from build123d import *

# Parameters (mm, degrees)
SKETCH_1_R           = 15
SKETCH_1_R_2         = 1.1
EXTRUDE_1_DEPTH      = 8
EXTRUDE_2_DEPTH      = 22
EXTRUDE_2_DEPTH_BACK = 22
SKETCH_5_W           = 12.455474759
SKETCH_5_H           = 13.140065833
CUT_EXTRUDE_1_DEPTH  = 15
CUT_EXTRUDE_START    = -15
CUT_EXTRUDE_2_DEPTH  = 15
SKETCH_7_R           = 4
EXTRUDE_3_DEPTH      = 2
SKETCH_8_R           = 3
CUT_EXTRUDE_3_DEPTH  = 1
DOME_1_FACE_RADIUS   = 3
DOME_1_HEIGHT        = 1.5
FILLET_1_R           = 3


with BuildPart() as part:
    # 草图1 → 凸台-拉伸1 (new body)
    with BuildSketch(Plane.XY):
        with BuildLine():
            Line((13.964240044, -17), (-13.964240044, -17))
            ThreePointArc((-13.964240044, -17), (-22, 0), (-13.964240044, 17))
            Line((-13.964240044, 17), (13.964240044, 17))
            ThreePointArc((13.964240044, 17), (22, 0), (13.964240044, -17))
        make_face()
        Circle(SKETCH_1_R, mode=Mode.SUBTRACT)
        with Locations((-13, 12)):
            Circle(SKETCH_1_R_2, mode=Mode.SUBTRACT)
        with Locations((13, 12)):
            Circle(SKETCH_1_R_2, mode=Mode.SUBTRACT)
        with Locations((13, -12)):
            Circle(SKETCH_1_R_2, mode=Mode.SUBTRACT)
        with Locations((-13, -12)):
            Circle(SKETCH_1_R_2, mode=Mode.SUBTRACT)
    extrude(amount=EXTRUDE_1_DEPTH)

    # 草图3 → 凸台-拉伸2 (add, two sides: drawn at the far end of the back side and taken through both)
    with BuildSketch(Plane(origin=(0, 0, 0), x_dir=(0, 0, -1), z_dir=(1, 0, 0)).offset(-EXTRUDE_2_DEPTH_BACK)):
        Polygon((-12, -6.8), (-12, -4.272567443), (-8, -1.093373368), (0, -1.093373368), (0, 6.340065833), (-8, 6.340065833), (-20.455474759, -3.559527056), (-20.455474759, -6.8), (-44, -6.8), (-44, -17), (-12, -17), align=None)
    extrude(amount=EXTRUDE_2_DEPTH + EXTRUDE_2_DEPTH_BACK)

    # 草图5 → 切除-拉伸1 (cut)
    with BuildSketch(Plane.ZY.offset(22)):
        with Locations((14.22773738, -0.229967084)):
            Rectangle(SKETCH_5_W, SKETCH_5_H)
    cut_extrude_1 = extrude(amount=-CUT_EXTRUDE_1_DEPTH, mode=Mode.SUBTRACT)

    # 镜向1: 切除-拉伸1 across plane
    add(cut_extrude_1.mirror(Plane(origin=(0, 0, 0), x_dir=(0, 0, 1), z_dir=(1, 0, 0))), mode=Mode.SUBTRACT)

    # 草图6 → 切除-拉伸2 (cut)
    with BuildSketch(Plane.XY.offset(8).offset(CUT_EXTRUDE_START)):
        with BuildLine():
            Line((21.066645799, 6.340065833), (22, 6.340065833))
            Line((22, 6.340065833), (22, 0))
            ThreePointArc((22, 0), (21.76541072, 3.204199776), (21.066645799, 6.340065833))
        make_face()
        with BuildLine():
            Line((-21.066645799, 6.340065833), (-22, 6.340065833))
            Line((-22, 6.340065833), (-22, 0))
            ThreePointArc((-22, 0), (-21.76541072, 3.204199776), (-21.066645799, 6.340065833))
        make_face()
    extrude(amount=CUT_EXTRUDE_2_DEPTH, mode=Mode.SUBTRACT)

    # 草图7 → 凸台-拉伸3 (add)
    with BuildSketch(Plane.XZ.offset(17)):
        with Locations(Location((0, 28, 0), (0, 0, 90))):
            Circle(SKETCH_7_R)
    extrude(amount=EXTRUDE_3_DEPTH)

    # 草图8 → 切除-拉伸3 (cut)
    with BuildSketch(Plane.XZ.offset(19)):
        with Locations(Location((0, 28, 0), (0, 0, 270))):
            Circle(SKETCH_8_R)
    extrude(amount=-CUT_EXTRUDE_3_DEPTH, mode=Mode.SUBTRACT)

    # 圆顶1: a dome of height H over a round flat face of radius A is a cap of a sphere of radius (A * A + H * H) / (2 * H)
    dome_1_r = (DOME_1_FACE_RADIUS * DOME_1_FACE_RADIUS + DOME_1_HEIGHT * DOME_1_HEIGHT) / (2 * DOME_1_HEIGHT)
    dome_1_base = Plane((0, -18, 28), z_dir=(0, -1, 0))
    with Locations(dome_1_base.offset(DOME_1_HEIGHT - dome_1_r)):
        dome_1_ball = Sphere(dome_1_r, mode=Mode.PRIVATE)
    add(split(dome_1_ball, bisect_by=dome_1_base, keep=Keep.TOP, mode=Mode.PRIVATE))

    # 圆角1
    fillet_1_edges = [part.edges().sort_by_distance(p)[0] for p in [
        (-22, -11.9, 12),
        (-22, -11.9, 44),
        (22, -11.9, 12),
        (22, -11.9, 44),
    ]]
    fillet(fillet_1_edges, radius=FILLET_1_R)


solid = part.part
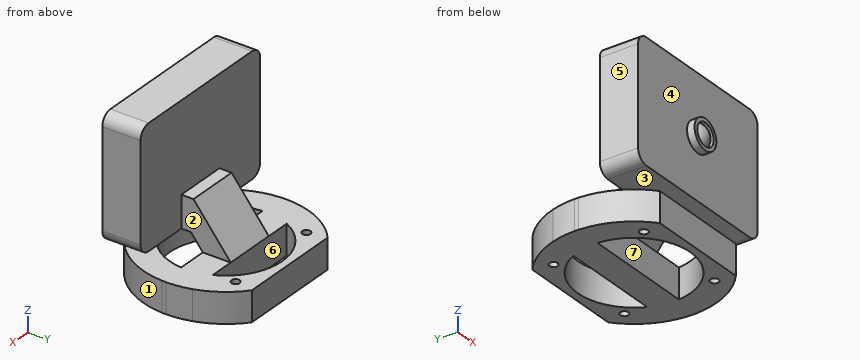
Build history of the part. All positions in model axes, mm. Face numbers are marked on the shaded views. A direction names the side the tool comes from. Round coordinates to 2 decimals unless told otherwise and drop trailing zeros. Write each loop counter-clockwise with the first axis right and the second up, starting at its lowest first coordinate (ties: lowest second). Pieces come first, ordered by that corner, then holes. Notation, with made-up numbers: M -15,58.25 L -1,58.25 A13 ccw -1,76.25 Z; hole C -5,40.5 d10. An arc over 180 degrees is marked long. Answer in a Markdown table with one row per item.
1. Saw through at A-A (x = 0). List the corners of the cut face in (y, z), and give its area (3 significant figures).
Geometry check:
| item | result |
|---|---|
| outline | M -19,24 L -17,24 L -17,12 L -4.27,12 L -1.09,8 L -1.09,0 L 6.34,0 L 6.34,8 L -3.56,20.46 L -6.8,20.46 L -6.8,44 L -17,44 L -17,32 L -19,32 L -19,31 L -18,31 A3.75 ccw -18,25 L -19,25 Z; M -17,0 L -15,0 L -15,8 L -17,8 Z; M 15,0 L 17,0 L 17,8 L 15,8 Z |
| area | 520 mm2 |
2. Probe L1, parallel to Z at x = 3.5, y = -16; L2, parallel to Y at x = 13, z = 2.75; L3, parallel to Z at x = 6, y = -4.5. List the from-to ranges inside material, lowest first. Write a range as [from, to].
Geometry check:
| item | result |
|---|---|
| L1 | [0, 8], [12, 44] |
| L2 | [-17, -13.1], [-10.9, -7.48], [-1.09, 6.34], [7.48, 10.9], [13.1, 17] |
| L3 | [12, 20.46] |
3. Which spindle directions (+Z, -Z, +X, -X, +Y, -Y) get a long thin tool onto all of the face, cutting with end or side? Do the marked faces 1, 2 and 3. Say none if no direction does.
Geometry check:
| item | result |
|---|---|
| face 1 | -Z, +X, -Y |
| face 2 | +Z, +X, +Y |
| face 3 | +X, -X, -Y |
4. Saw through at C-C (z = 4). State how many separate pieces and enclosed holes the cut face has, and give its area (3 significant figures).
Geometry check:
| item | result |
|---|---|
| separate pieces | 1 |
| enclosed holes | 6 |
| area | 825 mm2 |
5. Mould opens along X. For the marked faces 4, 5, 6 and 7 say: +X half, -X half, draft (parallel to the pull), parting line (faces both ways), or undercut.
Geometry check:
| item | result |
|---|---|
| face 4 | draft |
| face 5 | -X half |
| face 6 | undercut |
| face 7 | undercut |
6. Saw through at D-D (y = -12). List the corners of the cut face in (x, z), and give its area (3 significant figures).
Geometry check:
| item | result |
|---|---|
| outline | M -22,15 A3 ccw -19,12 L 19,12 A3 ccw 22,15 L 22,41 A3 ccw 19,44 L -19,44 A3 ccw -22,41 Z; M -18.44,0 L -14.1,0 L -14.1,8 L -18.44,8 Z; M -11.9,0 L -9,0 L -9,8 L -11.9,8 Z; M 9,0 L 11.9,0 L 11.9,8 L 9,8 Z; M 14.1,0 L 18.44,0 L 18.44,8 L 14.1,8 Z |
| area | 1,520 mm2 |
7. Saw through at B-B (y = 12). List the corners of the cut face in (x, z).
Geometry check:
| item | result |
|---|---|
| outline | M -18.44,0 L -14.1,0 L -14.1,8 L -18.44,8 Z; M -11.9,0 L -9,0 L -9,8 L -11.9,8 Z; M 9,0 L 11.9,0 L 11.9,8 L 9,8 Z; M 14.1,0 L 18.44,0 L 18.44,8 L 14.1,8 Z |
8. Flat gauge pins, fed straight in: P1, Ø8, axis at x = -9, z = 22, coming from the -Y side; P2, Ø6, axis at y = -1.5, z = 5.5, coming from the +X side; P3, Ø1, axis at x = 1, y = -5, coming from the +Z side; P4, Ø2, axis at x = 4, y = -4, coming from the -Z side. Where does each tip first touch, or does it go through?
Geometry check:
| item | result |
|---|---|
| P1 | y = -17 |
| P2 | x = 22 |
| P3 | z = 20.46 |
| P4 | z = 10.4 |
